Model file for the job. Use its own axes, mm. A direction names the side the tool comes from. Coordinates: 2 decimals unless noted, no trailing zeros. Loops run counter-clockwise (first coordinate to the right, second up) from the corner with the lowest first, then second, coordinate; pieces in that order, holes last. Notation, with made-up numbers: M -10,72.25 L 34,72.25 A25 ccw 34,91.25 Z; hole C -5,-18.75 d3. An arc over 180 degrees is marked long. One line per question, with ' | ' between items. Start each with the question number.
```python
from build123d import *

# Parameters (mm, degrees)
F1_DEPTH      = 25
F3_DEPTH      = 40.401
F3_DEPTH_BACK = 25
F4_R          = 1
F5_R          = 1


with BuildPart() as f1:
    # F0 (on Top) → F1 (new body)
    with BuildSketch(Plane.XY):
        Polygon((43.4, 0), (0, 0), (0, -48), (3, -48), (3, -3), (40.4, -3), (40.4, -48), (43.4, -48), align=None)
    extrude(amount=F1_DEPTH)

    # F2 (on face) → F3 (cut, two sides)
    with BuildSketch(Plane(origin=(40.4, 0, 0), x_dir=(0, -1, 0), z_dir=(-1, 0, 0))) as f3_sk:
        with BuildLine():
            Line((40.5, 12.5), (40.5, 15.1))
            ThreePointArc((40.5, 15.1), (37.9, 12.5), (40.5, 9.9))
            Line((40.5, 9.9), (40.5, 12.5))
        make_face()
        with BuildLine():
            ThreePointArc((43.1, 12.5), (42.338478, 14.338478), (40.5, 15.1))
            Line((40.5, 15.1), (40.5, 12.5))
            Line((40.5, 12.5), (40.5, 9.9))
            ThreePointArc((40.5, 9.9), (42.338478, 10.661522), (43.1, 12.5))
        make_face()
    extrude(amount=F3_DEPTH, mode=Mode.SUBTRACT)
    extrude(f3_sk.sketch, amount=-F3_DEPTH_BACK, mode=Mode.SUBTRACT)

    # F4
    f4_edges = [f1.edges().sort_by_distance(p)[0] for p in [
        (0, -48, 12.5),
        (3, -48, 12.5),
        (40.4, -48, 12.5),
        (43.4, -48, 12.5),
        (0, 0, 12.5),
    ]]
    fillet(f4_edges, radius=F4_R)

    # F5
    f5_edges = [f1.edges().sort_by_distance(p)[0] for p in [
        (43.4, 0, 12.5),
    ]]
    fillet(f5_edges, radius=F5_R)


solid = f1.part
```
(1) 3-axis set-ups, long thin cutter, end or side, ignore diameter. For faces 5 (the face through (3, -25, 12)), 6 (the face through (18.4, -2.6, 25)): which of +Z, -Z, +X, -X, +Y, -Y reach the whole face in a straight line?
(2) Band-saw the part on A-A on y = -26. Write the cut outline in (x, z), then the cut area to 3 significant figures.
(3) Two-plate mould, pull along X, no slides. Class faces 1 (the face through (0, -24, 12)), 2 (the face through (40.4, -25, 12)), 3 (the face through (18.4, -2.6, 0)), 4 (the face through (21, -3, 12)): pulls with the +X half, pulls with the -X half, needs draft (parallel to the pull), parting line crosses it, or undercut.
(4) Band-saw the part on B-B on z = 18. Write the cut outline in (x, y), then the cut area to 3 significant figures.
(5) Band-saw the part on C-C on z = 11.25. Write the cut outline in (x, y).
(6) Band-saw the part on D-D on x = 12. Write the cut outline in (y, z).
(7) Pin check, flat tip, straight feed: P1, Ø12.5, axis at x = 21, z = 10, coming from the -Y side. Stop position of the tip, or through.
(8) Drill centre lines: line 1 (X direction, y = -38, z = 23); line 2 (Y direction, x = 8, z = 22.75). Where is each one in solid material? Low to high. Write a range as [from, to].
Computed values:
1) face 5: +Z, -Z, -Y | face 6: +Z, +X, -X, +Y, -Y
2) outline: M 0,0 L 3,0 L 3,25 L 0,25 Z; M 40.4,0 L 43.4,0 L 43.4,25 L 40.4,25 Z | area: 150 mm^2
3) face 1: pulls with the -X half | face 2: undercut | face 3: needs draft | face 4: undercut
4) outline: M 0,-47 A1 ccw 1,-48 L 2,-48 A1 ccw 3,-47 L 3,-3 L 40.4,-3 L 40.4,-47 A1 ccw 41.4,-48 L 42.4,-48 A1 ccw 43.4,-47 L 43.4,-1 A1 ccw 42.4,0 L 1,0 A1 ccw 0,-1 Z | area: 399 mm^2
5) outline: M 0,-47 A1 ccw 1,-48 L 2,-48 A1 ccw 3,-47 L 3,-42.78 L 0,-42.78 Z; M 0,-38.22 L 3,-38.22 L 3,-3 L 40.4,-3 L 40.4,-38.22 L 43.4,-38.22 L 43.4,-1 A1 ccw 42.4,0 L 1,0 A1 ccw 0,-1 Z; M 40.4,-47 A1 ccw 41.4,-48 L 42.4,-48 A1 ccw 43.4,-47 L 43.4,-42.78 L 40.4,-42.78 Z
6) outline: M -3,0 L 0,0 L 0,25 L -3,25 Z
7) P1: y = -3
8) line 1: [0, 3], [40.4, 43.4] | line 2: [-3, 0]
